```python
from build123d import *

# Parameters (mm, degrees)
F0_R     = 11.43
F1_DEPTH = 6.35


with BuildPart() as f1:
    # F0 (on Top) → F1 (new body)
    with BuildSketch(Plane.XY):
        with BuildLine():
            Line((50.8, 0), (12.7, 0))
            ThreePointArc((12.7, 0), (3.719744, -3.719744), (0, -12.7))
            Line((0, -12.7), (0, -38.1))
            ThreePointArc((0, -38.1), (3.719744, -47.080256), (12.7, -50.8))
            Line((12.7, -50.8), (50.8, -50.8))
            Line((50.8, -50.8), (50.8, 0))
        make_face()
        with BuildLine():
            Line((101.6, 0), (50.8, 0))
            Line((50.8, 0), (50.8, -50.8))
            Line((50.8, -50.8), (101.6, -50.8))
            ThreePointArc((101.6, -50.8), (110.580256, -47.080256), (114.3, -38.1))
            Line((114.3, -38.1), (114.3, -12.7))
            ThreePointArc((114.3, -12.7), (110.580256, -3.719744), (101.6, 0))
        make_face()
        with Locations((82.55, -25.4)):
            Circle(F0_R, mode=Mode.SUBTRACT)
    extrude(amount=F1_DEPTH)


solid = f1.part
```
Work out the finished part from the listing and answer in its coordinate system (mm). Round coordinates to 2 decimals unless told otherwise and drop trailing zeros. Order: outer loops, then holes, each group sorted by start corner. A loop starts at its lowest first (then second) coordinate and runs counter-clockwise, first axis right, second up.
Q1. A cutting plane is placed at D-D, the plane x = 107. Determine the outline of the cut face in (y, z).
Solution:
outline: (-49.59, 0) - (-1.21, 0) - (-1.21, 6.35) - (-49.59, 6.35) - close
Q2. A cutting plane is placed at B-B, the plane x = 82.55. Determine the outline of the cut face in (y, z), then the cut area to 3 significant figures.
Solution:
outline: (-50.8, 0) - (-36.83, 0) - (-36.83, 6.35) - (-50.8, 6.35) - close; (-13.97, 0) - (0, 0) - (0, 6.35) - (-13.97, 6.35) - close
area: 177 mm2
Q3. Find the intervals of material crossed by line 1 along Y through (x, z) = (82.55, 4.75); line 2 along X through (y, z) = (-17, 1.5); line 3 along Y through (x, z) = (73.5, 3.75), in increasing order.
Solution:
line 1: y = -50.8 to -36.83, -13.97 to 0
line 2: x = 0 to 74.8, 90.3 to 114.3
line 3: y = -50.8 to -32.38, -18.42 to 0
Q4. Given pin 1 Ø10 at (x, y) = (62, -29.5) entering from -Z; pin 2 Ø1.5 at (y, z) = (-11, 3.5) entering from -X, each flat-ended and moving along its own axis, determine where each tip first touches the part or whether it passes through.
Solution:
pin 1: stops at z = 0
pin 2: stops at x = 0.04
Q5. A cutting plane is placed at C-C, the plane z = 2. Determine the outline of the cut face in (x, y), then the cut area to 3 significant figures.
Solution:
outline: (0, -38.1) arc R12.7 ccw to (12.7, -50.8) - (101.6, -50.8) arc R12.7 ccw to (114.3, -38.1) - (114.3, -12.7) arc R12.7 ccw to (101.6, 0) - (12.7, 0) arc R12.7 ccw to (0, -12.7) - close; hole circle Ø22.86 at (82.55, -25.4)
area: 5,260 mm2
Q6. A cutting plane is placed at A-A, the plane y = -25.4. Determine the outline of the cut face in (x, z).
Solution:
outline: (0, 0) - (71.12, 0) - (71.12, 6.35) - (0, 6.35) - close; (93.98, 0) - (114.3, 0) - (114.3, 6.35) - (93.98, 6.35) - close
Q7. The mould has two halves that part along X. Classify faces 1 (the flat face through (56, -25, 0)), 2 (the cylindrical face through (93.452, -21.967, 3.131)), 3 (the cylindrical face through (110.48, -47.18, 3.13)): pulls with the +X half, pulls with the -X half, needs draft (parallel to the pull), parting line crosses it, or undercut.
Solution:
face 1: needs draft
face 2: undercut
face 3: pulls with the +X half
